For this review, take the finished solid that the model builds, in its own axes (mm). Face numbers are marked on the shaded views. A direction names the side the tool comes from. Give positions to 0.01 mm unless a question says otherwise; leave off trailing zeros. Write each loop counter-clockwise with the first axis right and the second up, starting at its lowest first coordinate (ties: lowest second). Pieces come first, ordered by that corner, then holes.
Q1. We need section D-D (z = -9.5). Write out the cut boundary in (x, y).
Q2. Insertion check: P1, Ø5, axis at y = 4, z = -6.5, coming from the -X side; P2, Ø3, axis at x = -35.5, y = 4.5, coming from the -Z side; P3, Ø1.5, axis at x = -15.5, y = 3.5, coming from the +Z side. Each pin has a flat end and moves straight along its axis. Give the tip position at first contact, or say it passes through.
Q3. For line 1 (Z direction, x = -29, y = 7); line 2 (X direction, y = 0.75, z = -6); line 3 (X direction, y = 3.5, z = -27.5), list the stretches that pass through material, from the lowest coordinate up.
Q4. We need section A-A (x = -22). Write out the cut boundary in (y, z), then the cut area to 3 significant figures.
Q5. We need section C-C (z = -27). Write out the cut boundary in (x, y), then the cut area to 3 significant figures.
Q6. We need section B-B (y = 8.5). Write out the cut boundary in (x, z), then the cut area to 3 significant figures.
Q7. Machinability: for the marked faces 1, 2 and 3, which of the approach directions +Z, -Z, +X, -X, +Y, -Y give a long, thin tool a straight path to every point of the face, cutting with its end or side? Answer none if there is none.
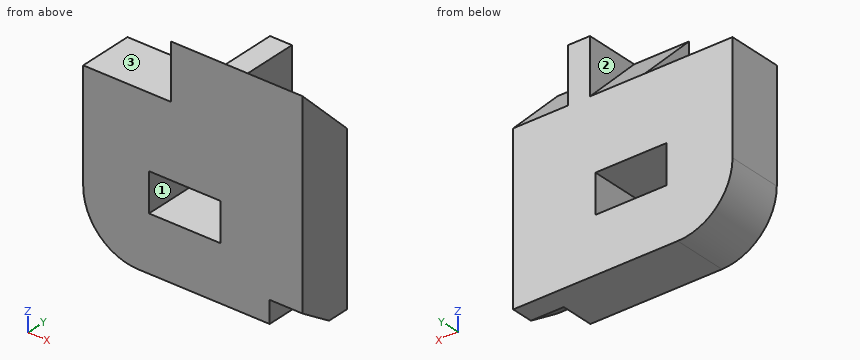
Autodesk Inventor part; units mm, degrees
ref_plane "YZ Plane" through (0, 0, 0) normal (1, 0, 0) x (0, 1, 0)
ref_plane "XZ Plane" through (0, 0, 0) normal (0, 1, 0) x (-1, 0, 0)
ref_plane "XY Plane" through (0, 0, 0) normal (0, 0, 1) x (1, 0, 0)
sketch "Sketch1" plane through (0, 0, 0) normal (0, 1, 0) x (-1, 0, 0)
  line L0 (0, 0) -> (10, 0)
  line L1 (10, 0) -> (14, 0)
  line L2 (14, 0) -> (24, 0)
  line L3 (24, 0) -> (24, -10)
  line L4 (24, -10) -> (40, -10)
  line L5 (0, 0) -> (0, -40)
  line L6 (0, -40) -> (30, -40)
  line L7 (40, -30) -> (40, -10)
  arc A0 (30, -40) -> (40, -30) centre (30, -30) ccw
  line L8 (28, -30) -> (15, -30)
  line L9 (15, -30) -> (15, -23)
  line L10 (15, -23) -> (28, -23)
  line L11 (28, -23) -> (28, -30)
  dimension "d0" = 10
  dimension "d1" = 4
  dimension "d2" = 10
  dimension "d3" = 10
  dimension "d4" = 16
  dimension "d5" = 40
  dimension "d6" = 10
  dimension "d7" = 13
  dimension "d8" = 7
  dimension "d9" = 13
  dimension "d10" = 12
extrude "Extrusion1" add sketch "Sketch1" along normal blind 10
sketch "Sketch2" plane through (-24, 0, -10) normal (-1, 0, 0) x (0, 0, 1)
  line L0 (0, 0) -> (0, 10)
  line L1 (-30, 0) -> (10, 0)
  line L2 (0, 10) -> (10, 0)
  line L3 (10, 0) -> (10, 10)
  line L4 (10, 10) -> (0, 10)
extrude "Extrusion2" cut sketch "Sketch2" against normal blind 10 contours L4 L3 L2
sketch "Sketch3" plane through (0, 0, 0) normal (1, 0, 0) x (0, 0, -1)
  line L0 (0, 0) -> (10, 10)
  line L1 (0, 0) -> (0, 10)
  line L2 (30, 10) -> (10, 10)
  line L3 (0, 0) -> (10, 10)
  line L4 (10, 10) -> (0, 10)
  line L5 (0, 10) -> (0, 0)
extrude "Extrusion3" cut sketch "Sketch3" against normal blind 10
sketch "Sketch4" plane through (0, 0, -40) normal (1, 0, 0) x (0, 0, -1)
  line L0 (0, 0) -> (-4, 0)
  line L1 (-10, 0) -> (0, 0)
  line L2 (0, 0) -> (0, 10)
  line L3 (0, 10) -> (0, 6)
  line L4 (0, 6) -> (-4, 0)
  line L5 (0, 6) -> (0, 0)
  point P0 (-40, 0)
  dimension "d17" = 4
  dimension "d18" = 4
extrude "Extrusion4" cut sketch "Sketch4" against normal blind 6
properties part number "T2 Part I"
Computed:
1. outline: (-24, 0) - (0, 0) - (0, 9.5) - (-10, 9.5) - (-10, 10) - (-14, 10) - (-14, 9.5) - (-24, 9.5) - close
2. P1: stops at x = -24
2. P2: stops at z = -39.17
2. P3: stops at z = -2.75
3. line 1: z = -40 to -10
3. line 2: x = -24 to 0
3. line 3: x = -40 to -28, -15 to 0
4. outline: (0, -40) - (10, -40) - (10, -30) - (0, -30) - close; (0, -23) - (10, -23) - (10, -10) - (0, 0) - close
4. area: 280 mm2
5. outline: (-40, 0) - (-28, 0) - (-28, 10) - (-40, 10) - close; (-15, 0) - (0, 0) - (0, 10) - (-15, 10) - close
5. area: 270 mm2
6. outline: (-40, -30) arc R10 ccw to (-30, -40) - (0, -40) - (0, -8.5) - (-10, -8.5) - (-10, 0) - (-14, 0) - (-14, -8.5) - (-24, -8.5) - (-24, -10) - (-40, -10) - close; hole (-28, -30) - (-15, -30) - (-15, -23) - (-28, -23) - close
6. area: 1,160 mm2
7. face 1: +Y, -Y
7. face 2: +Z, -X, +Y
7. face 3: +Z, -X, +Y, -Y
